Check sheet for the drawn part. Datum: minimum x, y, z corner. Units: mm. A direction names the side the tool comes from. Coordinates: 2 decimals unless noted, no trailing zeros. Order: outer loops, then holes, each group sorted by start corner. A loop starts at its lowest first (then second) coordinate and runs counter-clockwise, first axis right, second up.
Q1. Depth check by flat-ended pin: P1, Ø3, axis at x = 11.5, z = 5.5, coming from the -Y side; P2, Ø2, axis at x = 41, y = 7, coming from the +Z side; P3, Ø8, axis at x = 12.5, z = 10, coming from the +Y side. Enter the tip coordinate at first touch or a pass-through.
Q2. Cross-section at C-C, the plane x = 37. Record the boundary of the cut face in (y, z), and give its area (3 significant figures).
Q3. Cross-section at D-D, the plane z = 2. Record the boundary of the cut face in (x, y).
Q4. Set-up check for the marked faces 1 and 2: record each of +Z, -Z, +X, -X, +Y, -Y from which the full face is reachable in a straight line by a thin tool's end or side.
Q5. Cross-section at A-A, the plane z = 7. Record the boundary of the cut face in (x, y) (1 decimal).
Q6. Cross-section at B-B, the plane y = 7.25. Record the boundary of the cut face in (x, z) (1 decimal), and give its area (3 significant figures).
Q7. Thickness scan on line 1 (X direction, y = 3, z = 2); line 2 (Z direction, x = 35.5, y = 8); line 3 (Z direction, x = 26, y = 8.5). Record the ranges inside material, lowest first.
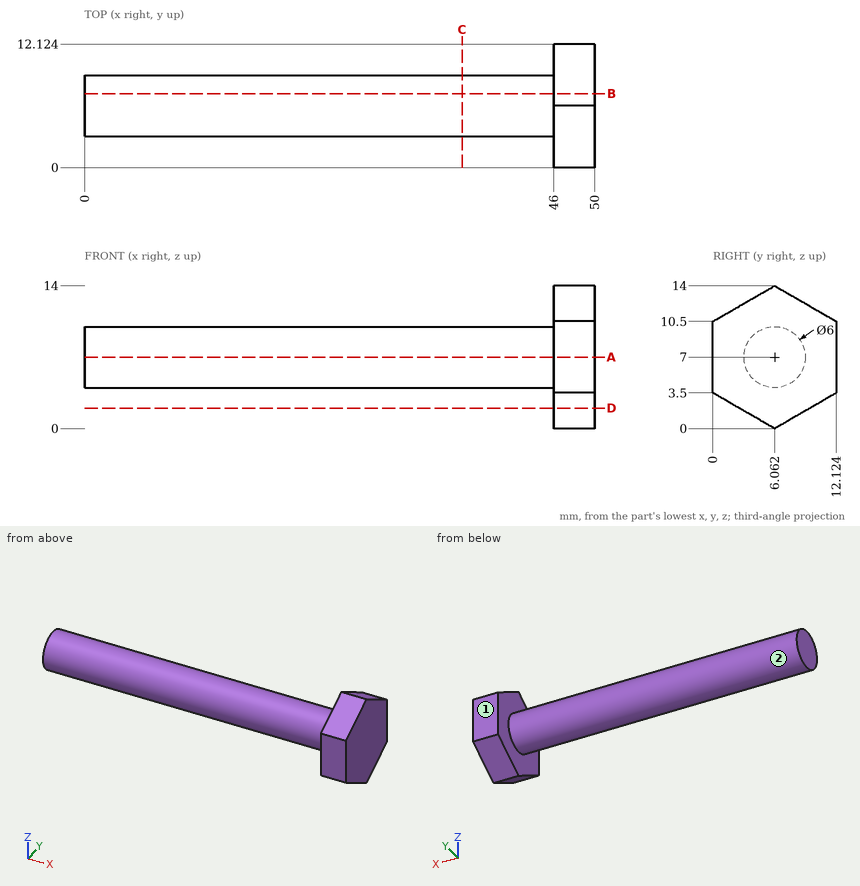
Check values:
1. P1: stops at y = 3.06
1. P2: stops at z = 10
1. P3: stops at y = 9.06
2. outline: circle Ø6 at (6.06, 7)
2. area: 28.3 mm2
3. outline: (46, 2.6) - (50, 2.6) - (50, 9.53) - (46, 9.53) - close
4. face 1: +Z, -Z, +X, -X, +Y
4. face 2: -X
5. outline: (0, 3.1) - (46, 3.1) - (46, 0) - (50, 0) - (50, 12.1) - (46, 12.1) - (46, 9.1) - (0, 9.1) - close
6. outline: (0, 4.2) - (46, 4.2) - (46, 0.7) - (50, 0.7) - (50, 13.3) - (46, 13.3) - (46, 9.8) - (0, 9.8) - close
6. area: 304 mm2
7. line 1: x = 46 to 50
7. line 2: z = 4.71 to 9.29
7. line 3: z = 5.25 to 8.75
